Can you work these out from the model? Positions are in its coordinate system, mm. Face numbers are marked on the shaded views. Coordinates: 2 decimals unless noted, no trailing zeros. Order: outer loops, then holes, each group sorted by start corner. A loop starts at its lowest first (then second) coordinate and runs counter-clockwise, first axis right, second up. Notation, with made-up numbers: M -6.5,-33 L 10.5,-33 A21 ccw 10.5,-11 Z; hole C -17,11.25 d10. An arc over 180 degrees is marked long. Answer as a JSON object with one key per item and string values.
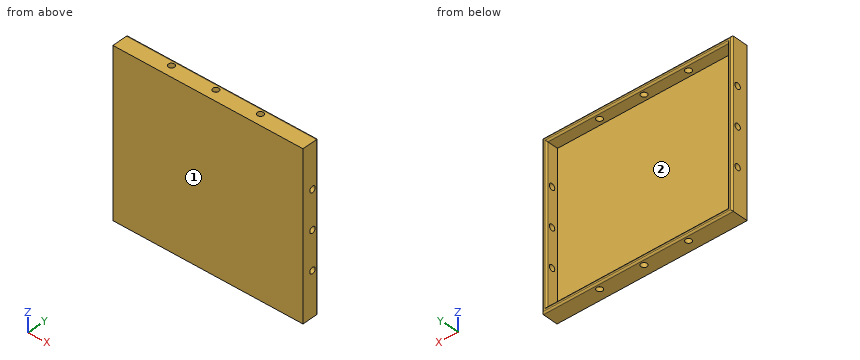
from build123d import *

# Parameters (mm, degrees)
SKETCH1_W               = 125
SKETCH1_H               = 108
BOSS_EXTRUDE1_DEPTH     = 11
SKETCH4_W               = 119
SKETCH4_H               = 102
CUT_EXTRUDE1_DEPTH      = 8
SKETCH6_R               = 2
CUT_EXTRUDE6_DEPTH      = 123
CUT_EXTRUDE6_DEPTH_BACK = 4
SKETCH5_R               = 2
CUT_EXTRUDE5_DEPTH      = 106
CUT_EXTRUDE5_DEPTH_BACK = 4
FILLET2_R               = 1


with BuildPart() as part:
    # Sketch1 → Boss-Extrude1 (new body)
    with BuildSketch(Plane(origin=(0, 0, 0), x_dir=(1, 0, 0), z_dir=(0, 1, 0))):
        with Locations((-139.109907121, 23.894736842)):
            Rectangle(SKETCH1_W, SKETCH1_H)
    extrude(amount=BOSS_EXTRUDE1_DEPTH)

    # Sketch4 → Cut-Extrude1 (cut)
    with BuildSketch(Plane(origin=(0, 11, 0), x_dir=(1, 0, 0), z_dir=(0, 1, 0))):
        with Locations((-139.109907121, 23.894736842)):
            Rectangle(SKETCH4_W, SKETCH4_H)
    extrude(amount=-CUT_EXTRUDE1_DEPTH, mode=Mode.SUBTRACT)

    # Sketch6 → Cut-Extrude6 (cut, two sides)
    with BuildSketch(Plane(origin=(-198.609907121, 0, 0), x_dir=(0, 0, -1), z_dir=(1, 0, 0))) as cut_extrude6_sk:
        with Locations((-1.105263158, 6.999999953)):
            Circle(SKETCH6_R)
        with Locations((23.894736842, 6.999999977)):
            Circle(SKETCH6_R)
        with Locations((48.894736842, 7)):
            Circle(SKETCH6_R)
    extrude(amount=CUT_EXTRUDE6_DEPTH, mode=Mode.SUBTRACT)
    extrude(cut_extrude6_sk.sketch, amount=-CUT_EXTRUDE6_DEPTH_BACK, mode=Mode.SUBTRACT)

    # Sketch5 → Cut-Extrude5 (cut, two sides)
    with BuildSketch(Plane.XY.offset(-74.894736842)) as cut_extrude5_sk:
        with Locations((-169.359907121, 7)):
            Circle(SKETCH5_R)
        with Locations((-140.109907121, 7)):
            Circle(SKETCH5_R)
        with Locations((-110.859907121, 7)):
            Circle(SKETCH5_R)
    extrude(amount=CUT_EXTRUDE5_DEPTH, mode=Mode.SUBTRACT)
    extrude(cut_extrude5_sk.sketch, amount=-CUT_EXTRUDE5_DEPTH_BACK, mode=Mode.SUBTRACT)

    # Fillet2
    fillet2_edges = [part.edges().sort_by_distance(p)[0] for p in [
        (-76.609907121, 11, -23.894736842),
        (-139.109907121, 11, -77.894736842),
        (-198.609907121, 11, -23.894736842),
        (-139.109907121, 11, 27.105263158),
        (-79.609907121, 11, -23.894736842),
        (-139.109907121, 11, -74.894736842),
        (-201.609907121, 11, -23.894736842),
        (-139.109907121, 11, 30.105263158),
    ]]
    fillet(fillet2_edges, radius=FILLET2_R)


solid = part.part
Item 1: I want a section at B-B, the plane x = -94.5. Write out the boundary of the cut face in (y, z).
Answers follow:
{"outline": "M 0,-77.89 L 10,-77.89 A1 ccw 11,-76.89 L 11,-75.89 A1 ccw 10,-74.89 L 3,-74.89 L 3,27.11 L 10,27.11 A1 ccw 11,28.11 L 11,29.11 A1 ccw 10,30.11 L 0,30.11 Z"}
Item 2: If we mould it in two halves opening along Z, with no side actions, what happens to the marked faces 1 and 2? For each: pulls with the +Z half, pulls with the -Z half, needs draft (parallel to the pull), parting line crosses it, or undercut.
Answers follow:
{"face 1": "needs draft", "face 2": "undercut"}
Item 3: I want a section at A-A, the plane z = 20. Write out the boundary of the cut face in (x, y), plus the area to 3 significant figures.
Answers follow:
{"outline": "M -201.61,0 L -76.61,0 L -76.61,10 A1 ccw -77.61,11 L -78.61,11 A1 ccw -79.61,10 L -79.61,3 L -198.61,3 L -198.61,10 A1 ccw -199.61,11 L -200.61,11 A1 ccw -201.61,10 Z", "area": "422 mm^2"}
Item 4: I want a section at C-C, the plane y = 7. Give the number of separate pieces and of enclosed holes in the cut face, plus the area to 3 significant figures.
Answers follow:
{"separate pieces": "12", "enclosed holes": "0", "area": "1,220 mm^2"}
Item 5: Please list where these lines run through material, in increasing order: line 1 (X direction, y = 7, z = 28.4); line 2 (Z direction, x = -187.5, y = 8.75); line 3 (X direction, y = 7, z = -63.5).
Answers follow:
{"line 1": "x = -201.61 to -171.36, -167.36 to -142.11, -138.11 to -112.86, -108.86 to -76.61", "line 2": "z = -77.89 to -74.89, 27.11 to 30.11", "line 3": "x = -201.61 to -198.61, -79.61 to -76.61"}
Item 6: I'm going to push flat-ended pins straight in: pin 1 (6 mm diameter, centred on x = -96.5, z = -55.5, fed in from +Y); pin 2 (3 mm diameter, centred on x = -110.86, y = 7, fed in from +Z). Where does each tip first touch, or does it pass through?
Answers follow:
{"pin 1": "stops at y = 3", "pin 2": "passes through"}
